Answer from the drawing. Dimensions are ordinates in mm from the lowest x, y and z of the part. A direction names the side the tool comes from. Round coordinates to 2 decimals unless told otherwise and drop trailing zeros. Write each loop counter-clockwise with the first axis right and the second up, starting at its lowest first coordinate (ties: lowest second). Pieces come first, ordered by that corner, then holes. Notation, with made-up numbers: M 71,84 L 110,84 A16 ccw 110,110 Z; hole C 66,-6.5 d1. An arc over 180 degrees is marked long. One line per item, written item: value. Start each with the question number.
(1) Section C-C (y = 183.5) is taken. Determine the outline of the cut face in (x, z).
(2) For a pull along X with two mould halves and no side action, classify the marked faces 1, 2 and 3 as released by +X, released by -X, zero draft, split by the parting line, or undercut.
(3) Given P1, Ø12, axis at x = 101, y = 225.5, coming from the +Z side; P2, Ø4, axis at x = 616, y = 340.5, coming from the -Z side, each flat-ended and moving along its own axis, determine where each tip first touches the part or whether it passes through.
(4) Section B-B (x = 296.5) is taken. Determine the outline of the cut face in (y, z), plus the area to 3 significant figures.
(5) Consider probe 1 along X at (y, z) = (318.5, 387.5); probe 2 along Z at (x, y) = (196.5, 150.5). Determine where each line is inside the solid, lowest interval first.
(6) For the marked faces 4, 5 and 6, determine the directions among +Z, -Z, +X, -X, +Y, -Y from which every point of the face is accessible in a straight line to the end or side of a thin tool.
(7) Section A-A (z = 614) is taken. Determine the outline of the cut face in (x, y).
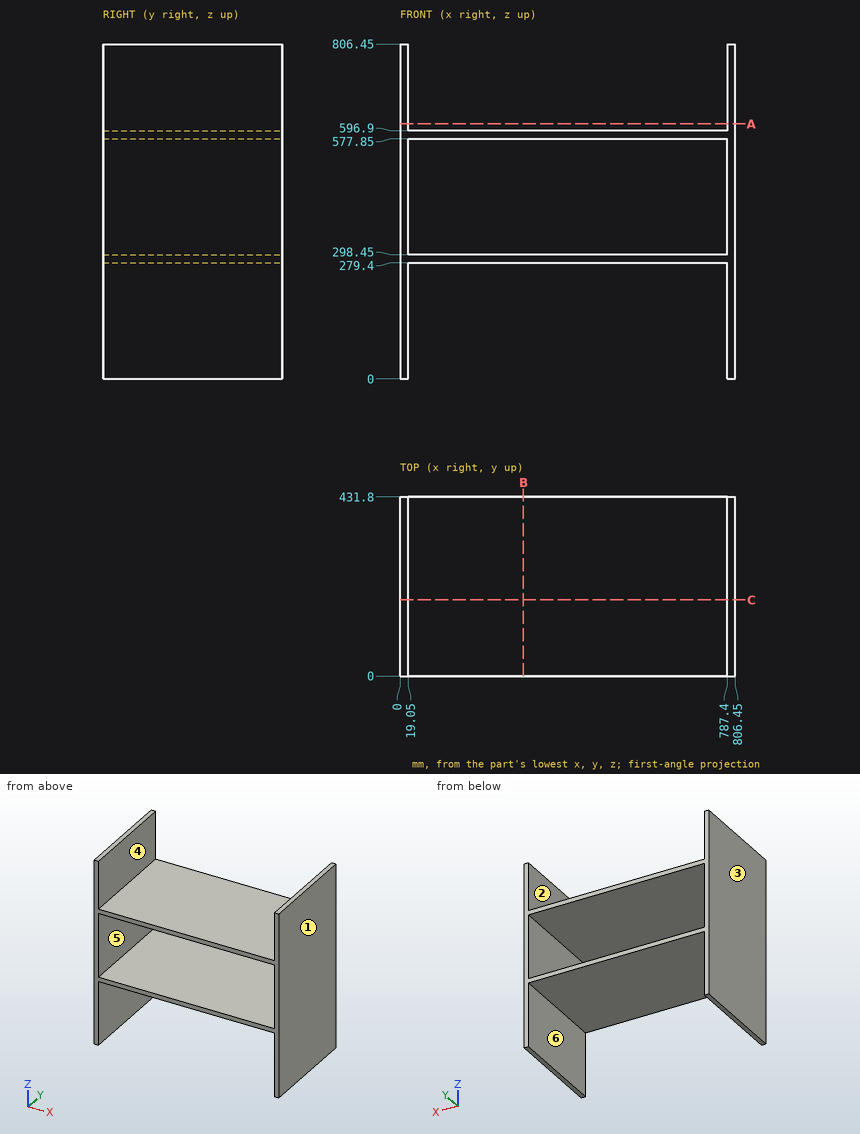
Recorded:
1. outline: M 0,0 L 19.05,0 L 19.05,279.4 L 787.4,279.4 L 787.4,0 L 806.45,0 L 806.45,806.45 L 787.4,806.45 L 787.4,596.9 L 19.05,596.9 L 19.05,806.45 L 0,806.45 Z; hole M 19.05,298.45 L 787.4,298.45 L 787.4,577.85 L 19.05,577.85 Z
2. face 1: released by +X
2. face 2: undercut
2. face 3: released by -X
3. P1: stops at z = 596.9
3. P2: stops at z = 279.4
4. outline: M 0,279.4 L 431.8,279.4 L 431.8,298.45 L 0,298.45 Z; M 0,577.85 L 431.8,577.85 L 431.8,596.9 L 0,596.9 Z
4. area: 16,500 mm2
5. probe 1: x = 0 to 19.05, 787.4 to 806.45
5. probe 2: z = 279.4 to 298.45, 577.85 to 596.9
6. face 4: +Z, +Y, -Y
6. face 5: +Y, -Y
6. face 6: -Z, +Y, -Y
7. outline: M 0,0 L 19.05,0 L 19.05,431.8 L 0,431.8 Z; M 787.4,0 L 806.45,0 L 806.45,431.8 L 787.4,431.8 Z
